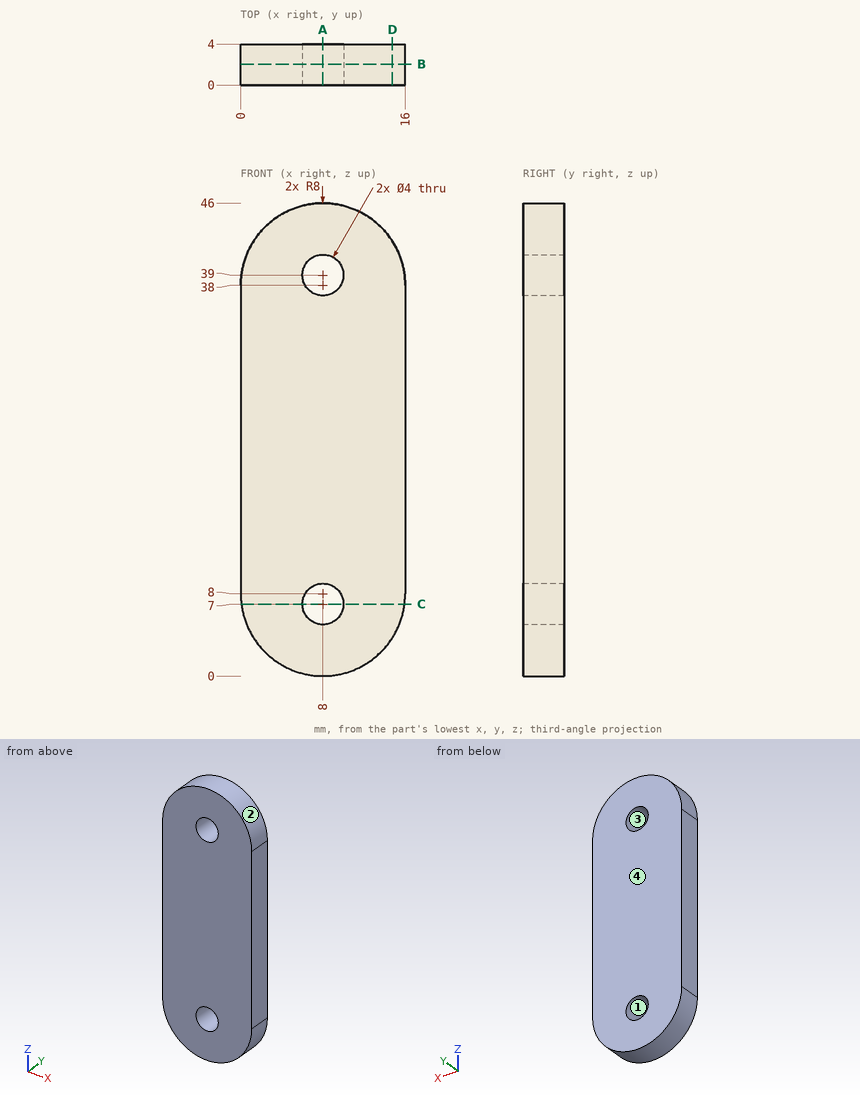
Geometry check sheet. Reference: drawing and pictorial views, mm from the part's lowest x, y, z. Round coordinates to 2 decimals unless told otherwise and drop trailing zeros. Loops run counter-clockwise (first coordinate to the right, second up) from the corner with the lowest first, then second, coordinate; pieces in that order, holes last. Notation, with made-up numbers: (-39.75, 17) -> (-2.75, 17) arc R22 ccw to (-2.75, 25) -> close; hole circle Ø11 at (84, -33). An arc over 180 degrees is marked (long way). Use a Markdown table: item, result.
(1) Sectioned sample at D-D (x = 14.75). Enter the section's corners in (y, z), then the cut area to 3 significant figures.
Calculated:
| item | result |
|---|---|
| outline | (0, 3.71) -> (4, 3.71) -> (4, 42.29) -> (0, 42.29) -> close |
| area | 154 mm² |
(2) Sectioned sample at B-B (y = 2.05). Enter the section's corners in (x, z).
Calculated:
| item | result |
|---|---|
| outline | (0, 8) arc R8 ccw to (16, 8) -> (16, 38) arc R8 ccw to (0, 38) -> close; hole circle Ø4 at (8, 7); hole circle Ø4 at (8, 39) |
(3) Scan lines: probe 1 along Z at (x, y) = (9.5, 3.4); probe 2 along X at (y, z) = (2.9, 7); probe 3 along X at (y, z) = (3.8, 4.5). Record each from-to range of solid material in increasing order.
Calculated:
| item | result |
|---|---|
| probe 1 | 0.14 to 5.68, 8.32 to 37.68, 40.32 to 45.86 |
| probe 2 | 0.06 to 6, 10 to 15.94 |
| probe 3 | 0.81 to 15.19 |
(4) Sectioned sample at A-A (x = 8). Enter the section's corners in (y, z), then the cut area to 3 significant figures.
Calculated:
| item | result |
|---|---|
| outline | (0, 0) -> (4, 0) -> (4, 5) -> (0, 5) -> close; (0, 9) -> (4, 9) -> (4, 37) -> (0, 37) -> close; (0, 41) -> (4, 41) -> (4, 46) -> (0, 46) -> close |
| area | 152 mm² |
(5) Mould release check, pull along Z, two halves, no side actions. Record for the marked faces 1, 2, 3 and 4: released by +Z, released by -Z, zero draft, split by the parting line, or undercut.
Calculated:
| item | result |
|---|---|
| face 1 | undercut |
| face 2 | released by +Z |
| face 3 | undercut |
| face 4 | zero draft |
(6) Sectioned sample at C-C (z = 7). Enter the section's corners in (x, y), then the cut area to 3 significant figures.
Calculated:
| item | result |
|---|---|
| outline | (0.06, 0) -> (6, 0) -> (6, 4) -> (0.06, 4) -> close; (10, 0) -> (15.94, 0) -> (15.94, 4) -> (10, 4) -> close |
| area | 47.5 mm² |
